from build123d import *

# Parameters (mm, degrees)
F1_DEPTH = 19
F3_W     = 25
F3_H     = 9
F4_DEPTH = 25
F5_R     = 3
F6_DEPTH = 5


with BuildPart() as f1:
    # F0 (on Front) → F1 (new body)
    with BuildSketch(Plane.XZ):
        Polygon((0, 30), (0, 0), (30, 0), (30, 5), (5, 30), align=None)
    extrude(amount=-F1_DEPTH)

    # F3 (on offset) → F4 (cut)
    with BuildSketch(Plane.XY.offset(30)):
        with Locations((17.5, 9.5)):
            Rectangle(F3_W, F3_H)
    extrude(amount=-F4_DEPTH, mode=Mode.SUBTRACT)

    # F5 (on face) → F6 (cut, through all)
    with BuildSketch(Plane(origin=(0, 0, 0), x_dir=(0, -1, 0), z_dir=(-1, 0, 0))):
        with Locations((-9.5, 20)):
            Circle(F5_R)
    extrude(amount=-F6_DEPTH, mode=Mode.SUBTRACT)


solid = f1.part
Can you work these out from the model? Positions are in its coordinate system, mm. A direction names the side the tool comes from. Give positions to 0.01 mm unless a question says otherwise; leave off trailing zeros. Write each loop counter-clockwise with the first axis right and the second up, starting at its lowest first coordinate (ties: lowest second). Pieces come first, ordered by that corner, then holes. Notation, with made-up numbers: M 83.25,11 L 122.25,11 A19 cw 122.25,35 Z; hole C 7,-28 d1. An arc over 180 degrees is marked long. Answer in a Markdown table with one row per item. Add a question column.
Item 1: Imagine slicing it at B-B, the plane y = 9.5. Write out the boundary of the cut face in (x, z).
Item 2: On a 3-axis mill with a long thin cutter (end or side, diameter ignored), from which of +Z, -Z, +X, -X, +Y, -Y can I reach the whole of each face in a straight line? I mean faces 1 (the flat face through (17, 10, 5)), 2 (the flat face through (3, 9, 30)). Say none if no direction works.
Item 3: We'd pull the mould along Y, two halves only. Please class faces 3 (the flat face through (0, 9, 15)), 4 (the flat face through (11, 0, 12)), 5 (the flat face through (5, 7, 18)): released by +Y, released by -Y, zero draft, split by the parting line, or undercut.
Item 4: Imagine slicing it at C-C, the plane x = 24. Write out the boundary of the cut face in (y, z), plus the area to 3 significant figures.
Item 5: Imagine slicing it at D-D, the plane z = 12. Write out the boundary of the cut face in (x, y).
Item 6: For pin 1 Ø4.5 at (x, y) = (23.5, 7.5) entering from +Z; pin 2 Ø5 at (y, z) = (9.5, 20) entering from +X; pin 3 Ø2.5 at (y, z) = (11, 23.5) entering from +X, each with a flat end and sliding along its axis, tell me the tip position at first contact or that it passes through.
Item 7: Imagine slicing it at A-A, the plane z = 20. Write out the boundary of the cut face in (x, y), plus the area to 3 significant figures.
Item 8: Please list where these lines run through material, in increasing order: L1, parallel to Z at x = 2.55, y = 9.5; L2, parallel to Y at x = 15.5, z = 10; L3, parallel to Z at x = 22.25, y = 6.25.
Evaluation:
| question | item | result |
|---|---|---|
| 1 | outline | M 0,0 L 30,0 L 30,5 L 5,5 L 5,17 L 0,17 Z; M 0,23 L 5,23 L 5,30 L 0,30 Z |
| 2 | face 1 | +Z, +X |
| 2 | face 2 | +Z, +X, -X, +Y, -Y |
| 3 | face 3 | zero draft |
| 3 | face 4 | released by -Y |
| 3 | face 5 | undercut |
| 4 | outline | M 0,0 L 19,0 L 19,11 L 14,11 L 14,5 L 5,5 L 5,11 L 0,11 Z |
| 4 | area | 155 mm² |
| 5 | outline | M 0,0 L 23,0 L 23,5 L 5,5 L 5,14 L 23,14 L 23,19 L 0,19 Z |
| 6 | pin 1 | stops at z = 5 |
| 6 | pin 2 | passes through |
| 6 | pin 3 | stops at x = 5 |
| 7 | outline | M 0,0 L 15,0 L 15,5 L 5,5 L 5,6.5 L 0,6.5 Z; M 0,12.5 L 5,12.5 L 5,14 L 15,14 L 15,19 L 0,19 Z |
| 7 | area | 165 mm² |
| 8 | L1 | z = 0 to 17, 23 to 30 |
| 8 | L2 | y = 0 to 5, 14 to 19 |
| 8 | L3 | z = 0 to 5 |
